```python
from build123d import *

# Parameters (mm, degrees)
SALIENTE_EXTRUIR1_DEPTH = 7
CROQUIS2_R              = 1.6
CORTAR_EXTRUIR1_DEPTH   = 6
CROQUIS3_R              = 2.75
CORTAR_EXTRUIR2_DEPTH   = 3


with BuildPart() as part:
    # Croquis1 → Saliente-Extruir1 (new body)
    with BuildSketch(Plane.XY):
        Polygon((0, 0), (7, 0), (10.5, 0), (10.5, 3.5), (0, 3.5), align=None)
    extrude(amount=SALIENTE_EXTRUIR1_DEPTH)

    # Croquis2 → Cortar-Extruir1 (cut)
    with BuildSketch(Plane.XZ):
        with Locations(Location((3.5, 3.5, 0), (0, 0, 270))):
            Circle(CROQUIS2_R)
    extrude(amount=-CORTAR_EXTRUIR1_DEPTH, mode=Mode.SUBTRACT)

    # Croquis3 → Cortar-Extruir2 (cut)
    with BuildSketch(Plane(origin=(0, 3.5, 0), x_dir=(1, 0, 0), z_dir=(0, 1, 0))):
        with Locations(Location((3.5, -3.5, 0), (0, 0, 180))):
            Circle(CROQUIS3_R)
    extrude(amount=-CORTAR_EXTRUIR2_DEPTH, mode=Mode.SUBTRACT)


solid = part.part
```
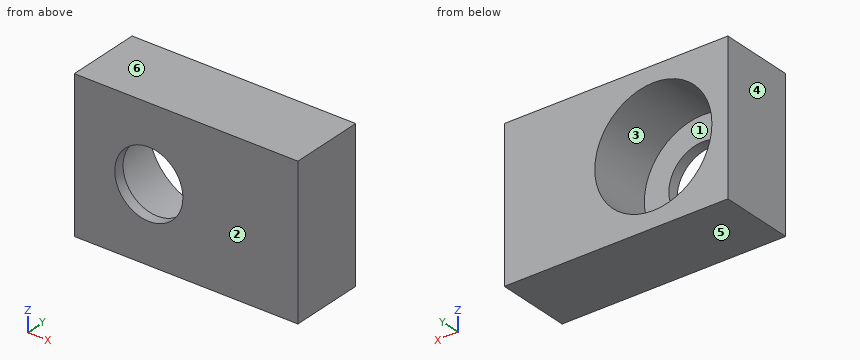
For this review, take the finished solid that the model builds, in its own axes (mm). Face numbers are marked on the shaded views. A direction names the side the tool comes from. Coordinates: 2 decimals unless noted, no trailing zeros. Order: outer loops, then holes, each group sorted by start corner. A loop starts at its lowest first (then second) coordinate and runs counter-clockwise, first axis right, second up. Notation, with made-up numbers: (-14, 78.25) - (12, 78.25) arc R15 ccw to (12, 87.25) - close; hole circle Ø1 at (47, 38.5). An arc over 180 degrees is marked (long way). Answer as a JSON object with one key per item and string values. Group by question number.
1. Clearance check with a flat-ended pin moving along its axis: P1, Ø1.5, axis at x = 6, z = 2.5, coming from the +Y side. State where the tip first meets the part, or that it passes through.
2. The part is to be moulded in two halves that separate along Z. For the marked faces 3, 4, 5 and 6, say which applies: pulls with the +Z half, pulls with the -Z half, needs draft (parallel to the pull), parting line crosses it, or undercut.
3. We need section B-B on z = 3.5. State the section outline as (x, y) points.
4. For the marked faces 1 and 2, list the 3-axis set-ups (+Z, -Z, +X, -X, +Y, -Y) from which the entire face can be reached by the end or side of a thin tool; tool diameter is ignored.
5. We need section A-A on x = 3.5. State the section outline as (y, z) points.
6. For probe 1 along X at (y, z) = (0.2, 3.5); probe 2 along Z at (x, y) = (3.5, 2.9); probe 3 along X at (y, z) = (2.25, 5), list the stretches that pass through material, from the lowest coordinate up.
7. We need section D-D on z = 1. State the section outline as (x, y) points.
8. We need section C-C on y = 1.2. State the section outline as (x, z) points, then the cut area to 3 significant figures.
Final values:
{
 "1": {"P1": "y = 3.5"},
 "2": {"face 3": "undercut", "face 4": "needs draft", "face 5": "pulls with the -Z half", "face 6": "pulls with the +Z half"},
 "3": {"outline": "(0, 0) - (1.9, 0) - (1.9, 0.5) - (0.75, 0.5) - (0.75, 3.5) - (0, 3.5) - close; (5.1, 0) - (10.5, 0) - (10.5, 3.5) - (6.25, 3.5) - (6.25, 0.5) - (5.1, 0.5) - close"},
 "4": {"face 1": "+Y", "face 2": "+Z, -Z, +X, -X, -Y"},
 "5": {"outline": "(0, 0) - (3.5, 0) - (3.5, 0.75) - (0.5, 0.75) - (0.5, 1.9) - (0, 1.9) - close; (0, 5.1) - (0.5, 5.1) - (0.5, 6.25) - (3.5, 6.25) - (3.5, 7) - (0, 7) - close"},
 "6": {"probe 1": "0 to 1.9, 5.1 to 10.5", "probe 2": "0 to 0.75, 6.25 to 7", "probe 3": "0 to 1.2, 5.8 to 10.5"},
 "7": {"outline": "(0, 0) - (10.5, 0) - (10.5, 3.5) - (4.65, 3.5) - (4.65, 0.5) - (2.35, 0.5) - (2.35, 3.5) - (0, 3.5) - close"},
 "8": {"outline": "(0, 0) - (10.5, 0) - (10.5, 7) - (0, 7) - close; hole circle Ø5.5 at (3.5, 3.5)", "area": "49.7 mm²"}
}
